For this review, take the finished solid that the model builds, in its own axes (mm). Give positions to 0.01 mm unless a question says otherwise; leave off trailing zeros. Write each loop counter-clockwise with the first axis right and the second up, starting at its lowest first coordinate (ties: lowest second). Pieces come first, ordered by that corner, then holes. Notation, with made-up numbers: M 9.25,-21 L 16.25,-21 A18 cw 16.25,-15 Z; hole C 60,19.5 d1. An arc over 180 degrees is marked long. Write item = value, one per line.
```python
from build123d import *

# Parameters (mm, degrees)
ESBO_O1_R          = 17.5
ESBO_O1_R_2        = 22.5
ESBO_O1_R_3        = 13
FLANGE_BASE1_DEPTH = 9.53


# Sheet-metal steps are written as plain solids
with BuildPart() as part:
    # Esboço1 → Flange-base1 (new body)
    with BuildSketch(Plane(origin=(0, 0, 0), x_dir=(0, 0, -1), z_dir=(1, 0, 0))):
        with BuildLine():
            Line((-40, 0), (-40, -95.693939399))
            ThreePointArc((-40, -95.693939399), (-55.649819015, -141.93282364), (-29.1335895, -182.918684903))
            Line((-29.1335895, -182.918684903), (60.212673691, -237.239402604))
            ThreePointArc((60.212673691, -237.239402604), (65.207688943, -239.408609141), (70.602684212, -240.15))
            Line((70.602684212, -240.15), (90, -240.15))
            Line((90, -240.15), (90, -230.15))
            Line((90, -230.15), (140, -230.15))
            Line((140, -230.15), (140, -184.65))
            Line((140, -184.65), (90, -184.65))
            Line((90, -184.65), (90, -174.65))
            Line((90, -174.65), (140, -174.65))
            Line((140, -174.65), (140, 0))
            Line((140, 0), (56.568542495, 0))
            ThreePointArc((56.568542495, 0), (45.021537111, 3.670068381), (37.712361663, 13.333333333))
            ThreePointArc((37.712361663, 13.333333333), (-6.764079149, 39.423942386), (-40, 0))
        make_face()
        Circle(ESBO_O1_R, mode=Mode.SUBTRACT)
        with Locations((0, -135)):
            Circle(ESBO_O1_R_2, mode=Mode.SUBTRACT)
        with Locations((49.01, -33)):
            Circle(ESBO_O1_R_3, mode=Mode.SUBTRACT)
    extrude(amount=-FLANGE_BASE1_DEPTH)


solid = part.part
```
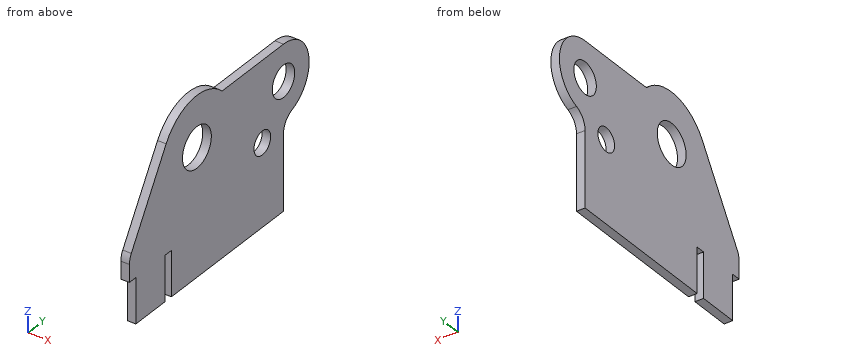
1. We need section C-C, the plane z = 0. Write out the cut boundary in (x, y), then the cut area to 3 significant figures.
Responses:
outline = M -9.53,-200.63 L 0,-200.63 L 0,-157.5 L -9.53,-157.5 Z; M -9.53,-112.5 L 0,-112.5 L 0,-17.5 L -9.53,-17.5 Z; M -9.53,17.5 L 0,17.5 L 0,40 L -9.53,40 Z
area = 1,530 mm2
2. We need section A-A, the plane y = -135. Write out the cut boundary in (x, z), then the cut area to 3 significant figures.
Responses:
outline = M -9.53,-140 L 0,-140 L 0,-22.5 L -9.53,-22.5 Z; M -9.53,22.5 L 0,22.5 L 0,56.08 L -9.53,56.08 Z
area = 1,440 mm2
3. We need section D-D, the plane z = -49.01. Write out the cut boundary in (x, y).
Responses:
outline = M -9.53,-230.43 L 0,-230.43 L 0,-46 L -9.53,-46 Z; M -9.53,-20 L 0,-20 L 0,1.48 L -9.53,1.48 Z
4. We need section B-B, the plane x = -1.75. Write out the cut boundary in (y, z).
Responses:
outline = M -240.15,-90 L -230.15,-90 L -230.15,-140 L -184.65,-140 L -184.65,-90 L -174.65,-90 L -174.65,-140 L 0,-140 L 0,-56.57 A20 cw 13.33,-37.71 A40 ccw 0,40 L -95.69,40 A56.08 ccw -182.92,29.13 L -237.24,-60.21 A20 ccw -240.15,-70.6 Z; hole C -135,0 d45; hole C -33,-49.01 d26; hole C 0,0 d35
5. For line 1 along Y through (x, z) = (-8, -101); line 2 along Y through (x, z) = (-4, 0); line 3 along Y through (x, z) = (-8.25, 1), list the stretches that pass through material, from the lowest coordinate up. Write a range as from..to.
Responses:
line_1 = -230.15..-184.65, -174.65..0
line_2 = -200.63..-157.5, -112.5..-17.5, 17.5..40
line_3 = -200.02..-157.48, -112.52..-17.47, 17.47..39.99
6. Insertion check: P1, Ø6, axis at y = -2.5, z = 13, coming from the +X side; P2, Ø3, axis at x = -6, y = -162, coming from the +Z side; P3, Ø3, axis at x = -5, y = -235, coming from the -Z side; P4, Ø1.5, axis at y = -68, z = -49, coming from the +X side. Each pin has a flat end and moves straight along its axis. Give the tip position at first contact, or say it passes through.
Responses:
P1 = through
P2 = 49.95
P3 = -90
P4 = 0
